The listing builds one solid part. Answer for the finished solid, in the listing's coordinates (mm). A direction names the side the tool comes from. Give positions to 0.01 mm unless a question says otherwise; leave off trailing zeros. Write each loop counter-clockwise with the first axis right and the second up, starting at its lowest first coordinate (ties: lowest second). Pieces come first, ordered by that corner, then holes. Notation, with made-up numbers: (81, 80) - (123, 80) arc R18 ccw to (123, 109) - close; hole circle Ø9 at (7, 48.5). An arc over 180 degrees is marked (long way). One line per question, with ' | ' between items. Start each with the question number.
1. A cutting plane is placed at A-A (x = 90.5). Determine the outline of the cut face in (y, z), then the cut area to 3 significant figures.
2. The mould has two halves that part along Y. Classify faces 3 (the face through (177.8, 97, 16)), 4 (the face through (97, 196.85, 16)), 5 (the face through (97, 19.05, 16)), 6 (the face through (196.85, 97, 16)): +Y half, -Y half, draft (parallel to the pull), parting line (faces both ways), or undercut.
3. Find the intervals of material crossed by L1, parallel to Y at x = 118.5, z = 26, in increasing order. Write a range as from..to.
4. For faces 1 (the face through (97, 0, 16)), 2 (the face through (19.05, 97, 16)), determine the directions among +Z, -Z, +X, -X, +Y, -Y from which every point of the face is accessible in a straight line to the end or side of a thin tool.
5. A cutting plane is placed at C-C (z = 28). Determine the outline of the cut face in (x, y) (3 decimals).
```python
from build123d import *

# Parameters (mm, degrees)
SKETCH001_R      = 2
EXTRUDE001_DEPTH = 40
SKETCH_W         = 196.85
SKETCH_H         = 196.85
SKETCH_W_2       = 158.75
SKETCH_H_2       = 158.75
EXTRUDE_DEPTH    = 33.02


with BuildPart() as extrude001:
    # Sketch001 (on Face10 of Extrude) → Extrude001 (new body)
    with BuildSketch(Plane.XY.offset(33.02)):
        with Locations((9.525, 187.325)):
            Circle(SKETCH001_R)
        with Locations((187.325, 187.325)):
            Circle(SKETCH001_R)
        with Locations((187.325, 9.525)):
            Circle(SKETCH001_R)
        with Locations((9.525, 9.525)):
            Circle(SKETCH001_R)
    extrude(amount=-EXTRUDE001_DEPTH)


with BuildPart() as wall:
    # Sketch → Extrude (new body)
    with BuildSketch(Plane.XY):
        with Locations((98.425, 98.425)):
            Rectangle(SKETCH_W, SKETCH_H)
        with Locations((98.425, 98.425)):
            Rectangle(SKETCH_W_2, SKETCH_H_2, mode=Mode.SUBTRACT)
    extrude(amount=EXTRUDE_DEPTH)

    # Cut: cut Extrude001
    add(extrude001.part, mode=Mode.SUBTRACT)


solid = wall.part
```
Determined:
1) outline: (0, 0) - (19.05, 0) - (19.05, 33.02) - (0, 33.02) - close; (177.8, 0) - (196.85, 0) - (196.85, 33.02) - (177.8, 33.02) - close | area: 1,260 mm2
2) face 3: undercut | face 4: +Y half | face 5: undercut | face 6: draft
3) L1: 0..19.05, 177.8..196.85
4) face 1: +Z, -Z, +X, -X, -Y | face 2: +Z, -Z
5) outline: (0, 0) - (196.85, 0) - (196.85, 196.85) - (0, 196.85) - close; hole circle Ø4 at (9.525, 9.525); hole circle Ø4 at (9.525, 187.325); hole (19.05, 19.05) - (177.8, 19.05) - (177.8, 177.8) - (19.05, 177.8) - close; hole circle Ø4 at (187.325, 9.525); hole circle Ø4 at (187.325, 187.325)
